Build history of the part. All positions in model axes, mm. Face numbers are marked on the shaded views. A direction names the side the tool comes from. Give positions to 0.01 mm unless a question says otherwise; leave off trailing zeros. Order: outer loops, then holes, each group sorted by start corner. A loop starts at its lowest first (then second) coordinate and runs counter-clockwise, first axis right, second up. Notation, with made-up numbers: (84.5, 66) - (102.5, 66) arc R9 cw to (102.5, 77) - close; hole circle Ø6 at (50, 75.5). An arc over 180 degrees is marked (long way). Use a Markdown table: item, result.
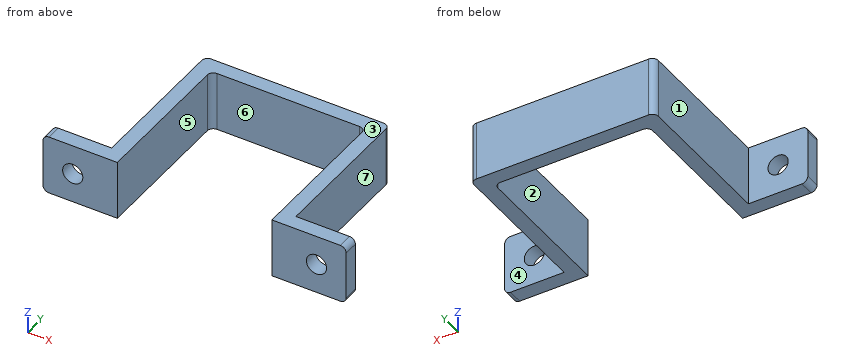
from build123d import *

# Parameters (mm, degrees)
BOSS_EXTRUDE1_DEPTH   = 12.7
F_6_CLEARANCE_HOLE1_D = 4.3053
FILLET1_R             = 1.27


with BuildPart() as part:
    # Sketch1 → Boss-Extrude1 (new body)
    with BuildSketch(Plane.XY):
        Polygon((-15.875, 0), (0, 0), (0, 32.385), (33.02, 32.385), (33.02, 0), (48.895, 0), (48.895, 3.175), (36.195, 3.175), (36.195, 35.56), (-3.175, 35.56), (-3.175, 3.175), (-15.875, 3.175), align=None)
    extrude(amount=BOSS_EXTRUDE1_DEPTH)

    # #6 Clearance Hole1 (through all)
    with Locations(Plane(origin=(0, 3.175, 0), x_dir=(1, 0, 0), z_dir=(0, 1, 0))):
        with Locations((-9.525, -6.35), (42.545, -6.35)):
            Hole(F_6_CLEARANCE_HOLE1_D / 2)

    # Fillet1
    fillet1_edges = [part.edges().sort_by_distance(p)[0] for p in [
        (48.895, 1.5875, 0),
        (-15.875, 1.5875, 0),
        (-3.175, 35.56, 6.35),
        (36.195, 35.56, 6.35),
        (33.02, 32.385, 6.35),
        (0, 32.385, 6.35),
        (48.895, 1.5875, 12.7),
        (-15.875, 1.5875, 12.7),
    ]]
    fillet(fillet1_edges, radius=FILLET1_R)


solid = part.part
1) Slice it at A-A (y = 18). Write the cut outline in (x, z) (3 decimals).
Computed:
| item | result |
|---|---|
| outline | (-3.175, 0) - (0, 0) - (0, 12.7) - (-3.175, 12.7) - close; (33.02, 0) - (36.195, 0) - (36.195, 12.7) - (33.02, 12.7) - close |
2) Slice it at B-B (z = 6.35). Write the cut outline in (x, y) (3 decimals).
Computed:
| item | result |
|---|---|
| outline | (-15.875, 0) - (-11.678, 0) - (-11.678, 3.175) - (-15.875, 3.175) - close; (-7.372, 0) - (0, 0) - (0, 31.115) arc R1.27 cw to (1.27, 32.385) - (31.75, 32.385) arc R1.27 cw to (33.02, 31.115) - (33.02, 0) - (40.392, 0) - (40.392, 3.175) - (36.195, 3.175) - (36.195, 34.29) arc R1.27 ccw to (34.925, 35.56) - (-1.905, 35.56) arc R1.27 ccw to (-3.175, 34.29) - (-3.175, 3.175) - (-7.372, 3.175) - close; (44.698, 0) - (48.895, 0) - (48.895, 3.175) - (44.698, 3.175) - close |
3) Two-plate mould, pull along X, no slides. Class the marked faces 4, 5, 6 and 7: +X half, -X half, draft (parallel to the pull), parting line (faces both ways), or undercut.
Computed:
| item | result |
|---|---|
| face 4 | draft |
| face 5 | undercut |
| face 6 | undercut |
| face 7 | +X half |
4) Slice it at D-D (x = 11.5). Write the cut outline in (y, z) (3 decimals).
Computed:
| item | result |
|---|---|
| outline | (32.385, 0) - (35.56, 0) - (35.56, 12.7) - (32.385, 12.7) - close |
5) Wall check: line 1 (X direction, y = 4.5, z = 4.5) (3 decimals); line 2 (Y direction, x = 22, z = 1.5) (3 decimals); line 3 (Y direction, x = 41, z = 11.25) (3 decimals). Give the ranges that are in metal, low to high. Write a range as from..to.
Computed:
| item | result |
|---|---|
| line 1 | x = -3.175..0, 33.02..36.195 |
| line 2 | y = 32.385..35.56 |
| line 3 | y = 0..3.175 |
6) Slice it at C-C (z = 3.25). Write the cut outline in (x, y) (3 decimals), and give its area (3 significant figures).
Computed:
| item | result |
|---|---|
| outline | (-15.875, 0) - (0, 0) - (0, 31.115) arc R1.27 cw to (1.27, 32.385) - (31.75, 32.385) arc R1.27 cw to (33.02, 31.115) - (33.02, 0) - (48.895, 0) - (48.895, 3.175) - (36.195, 3.175) - (36.195, 34.29) arc R1.27 ccw to (34.925, 35.56) - (-1.905, 35.56) arc R1.27 ccw to (-3.175, 34.29) - (-3.175, 3.175) - (-15.875, 3.175) - close |
| area | 411 mm² |
7) Pin check, flat tips, straight feed: P1, Ø4, axis at x = 18.5, z = 8, coming from the -Y side (3 decimals); P2, Ø5, axis at y = 18, z = 3.5, coming from the +X side (3 decimals); P3, Ø4, axis at y = 19, z = 4.5, coming from the -X side (3 decimals). Stop position of each tip, or through.
Computed:
| item | result |
|---|---|
| P1 | stops at y = 32.385 |
| P2 | stops at x = 36.195 |
| P3 | stops at x = -3.175 |
8) Tool access for the marked faces 1, 2 and 3: list every direction of +Z, -Z, +X, -X, +Y, -Y with a clear straight run to the whole face (end or side of a thin tool).
Computed:
| item | result |
|---|---|
| face 1 | +Z, -Z, -X, +Y |
| face 2 | +Z, -Z, -Y |
| face 3 | +Z, +X, -X, +Y, -Y |
